Geometry check sheet. Reference: the model listing, model coordinates, mm. Round coordinates to 2 decimals unless told otherwise and drop trailing zeros. Write each loop counter-clockwise with the first axis right and the second up, starting at its lowest first coordinate (ties: lowest second). Pieces come first, ordered by that corner, then holes. Notation, with made-up numbers: M 60.25,37 L 104.25,37 A18 ccw 104.25,68 Z; hole C 53,-30.75 d9. An arc over 180 degrees is marked long. Use a Markdown table: item, result.
```python
from build123d import *

# Parameters (mm, degrees)
BOSS_EXTRU_1_DEPTH      = 2
ESQUISSE4_R             = 0.75
ENL_V_MAT_EXTRU_2_DEPTH = 176.894862906
ENL_V_MAT_EXTRU_3_DEPTH = 4
CONG_2_R                = 1.35
ESQUISSE12_W            = 2
ESQUISSE12_H            = 5
BOSS_EXTRU_2_DEPTH      = 3


with BuildPart() as part:
    # Esquisse2 → Boss.-Extru.1 (new body)
    with BuildSketch(Plane(origin=(0, 0, 0), x_dir=(0, 0, -1), z_dir=(1, 0, 0))):
        with BuildLine():
            Line((0, 0), (170.873171093, 0))
            ThreePointArc((170.873171093, 0), (174.177922559, 2.347343181), (173.049882129, 6.240789861))
            ThreePointArc((173.049882129, 6.240789861), (150.444362328, 18.689979585), (125, 23))
            ThreePointArc((125, 23), (61.450806457, 17.202138822), (0, 0))
        make_face()
    extrude(amount=BOSS_EXTRU_1_DEPTH)

    # Esquisse4 → Enlèv. mat.-Extru.2 (cut, through all)
    with BuildSketch(Plane(origin=(2, 0, 0), x_dir=(0, 0, -1), z_dir=(1, 0, 0))):
        with Locations((125, 21.75)):
            Circle(ESQUISSE4_R)
        with Locations((172.618958832, 3.328337296)):
            Circle(ESQUISSE4_R)
        with Locations((8, 1.25)):
            Circle(ESQUISSE4_R)
    extrude(amount=-ENL_V_MAT_EXTRU_2_DEPTH, mode=Mode.SUBTRACT)

    # Esquisse9 → Enlèv. mat.-Extru.3 (cut)
    with BuildSketch(Plane(origin=(0, 0, 0), x_dir=(0, 0, -1), z_dir=(1, 0, 0))):
        with BuildLine():
            Line((126, 1.5), (170.873171093, 1.5))
            ThreePointArc((170.873171093, 1.5), (171.378747106, 1.564956617), (171.851482612, 1.755607106))
            ThreePointArc((171.851482612, 1.755607106), (170.877358103, 3.499588293), (172.172511728, 5.020432147))
            ThreePointArc((172.172511728, 5.020432147), (172.144964437, 5.043548409), (172.11700597, 5.066165635))
            ThreePointArc((172.11700597, 5.066165635), (150.432293025, 17.103742315), (126.021977416, 21.493106696))
            ThreePointArc((126.021977416, 21.493106696), (126.011314857, 21.467285013), (126, 21.441742431))
            Line((126, 21.441742431), (126, 1.5))
        make_face()
        with BuildLine():
            Line((9.071214264, 1.5), (60, 1.5))
            Line((60, 1.5), (60, 15.405547145))
            ThreePointArc((60, 15.405547145), (34.242807282, 9.516740415), (9.003792697, 1.699889121))
            ThreePointArc((9.003792697, 1.699889121), (9.042306283, 1.601564521), (9.071214264, 1.5))
        make_face()
        with BuildLine():
            Line((124, 21.441742431), (124, 1.5))
            Line((124, 1.5), (61.5, 1.5))
            Line((61.5, 1.5), (61.5, 15.685935533))
            ThreePointArc((61.5, 15.685935533), (92.607306096, 19.996388454), (123.975891605, 21.498500317))
            ThreePointArc((123.975891605, 21.498500317), (123.987547995, 21.469952401), (124, 21.441742431))
        make_face()
    extrude(amount=ENL_V_MAT_EXTRU_3_DEPTH, mode=Mode.SUBTRACT)

    # Congé2
    cong_2_edges = [part.edges().sort_by_distance(p)[0] for p in [
        (1, 0, 0),
    ]]
    fillet(cong_2_edges, radius=CONG_2_R)

    # Esquisse12 → Boss.-Extru.2 (add)
    with BuildSketch(Plane.XZ):
        with Locations((1, -138.373171093)):
            Rectangle(ESQUISSE12_W, ESQUISSE12_H)
        with Locations((1, -43.373171093)):
            Rectangle(ESQUISSE12_W, ESQUISSE12_H)
    extrude(amount=BOSS_EXTRU_2_DEPTH)


solid = part.part
```
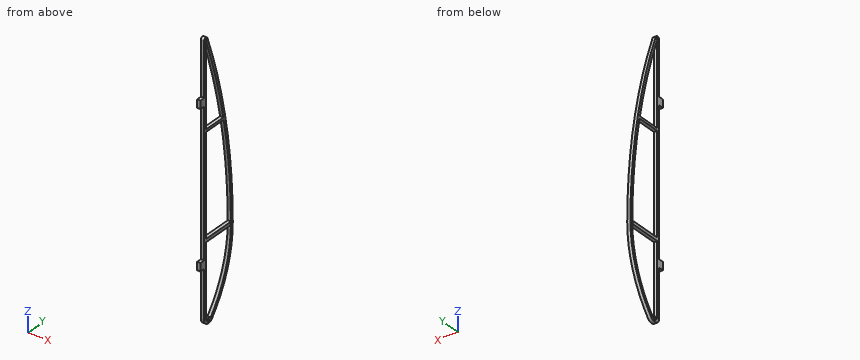
Item 1: Cross-section at C-C, the plane x = 0.5. Count the separate pieces of the cut face and the enclosed holes in it, and give its area (3 significant figures).
Outcome:
| item | result |
|---|---|
| separate pieces | 1 |
| enclosed holes | 6 |
| area | 605 mm2 |
Item 2: Go/stop test with flat-tipped pins: pin 1 (1 mm diameter, centred on x = 1, y = 7, fed in from -Z); pin 2 (1 mm diameter, centred on x = 1, z = -135, fed in from -Y); pin 3 (8 mm diameter, centred on y = 16, z = -99.5, fed in from -X); pin 4 (0.6 mm diameter, centred on x = 1, y = -2, fed in from +Z). Record where each tip stops, or that it passes through.
Outcome:
| item | result |
|---|---|
| pin 1 | stops at z = -172.72 |
| pin 2 | stops at y = 0 |
| pin 3 | passes through |
| pin 4 | stops at z = -40.87 |
Item 3: Cross-section at B-B, the plane y = 11.75. Record the cut outline in (x, z).
Outcome:
| item | result |
|---|---|
| outline | M 0,-165.15 L 2,-165.15 L 2,-162.18 L 0,-162.18 Z; M 0,-126 L 2,-126 L 2,-124 L 0,-124 Z; M 0,-61.5 L 2,-61.5 L 2,-60 L 0,-60 Z; M 0,-43 L 2,-43 L 2,-36.82 L 0,-36.82 Z |
Item 4: Cross-section at A-A, the plane y = 19. Record the cut outline in (x, z).
Outcome:
| item | result |
|---|---|
| outline | M 0,-149.54 L 2,-149.54 L 2,-144.3 L 0,-144.3 Z; M 0,-126 L 2,-126 L 2,-124 L 0,-124 Z; M 0,-83.26 L 2,-83.26 L 2,-72.15 L 0,-72.15 Z |
Item 5: Material ranges on line 1 along Y through (x, z) = (1, -125); line 2 along Y through (x, z) = (1.45, -152.5); line 3 along Z through (x, y) = (1.7, 0.75), recorded low to high. Write a range as from..to.
Outcome:
| item | result |
|---|---|
| line 1 | y = 0..21, 22.5..23 |
| line 2 | y = 0..1.5, 16.33..17.94 |
| line 3 | z = -173.04..-8.56, -7.44..-6.36 |
